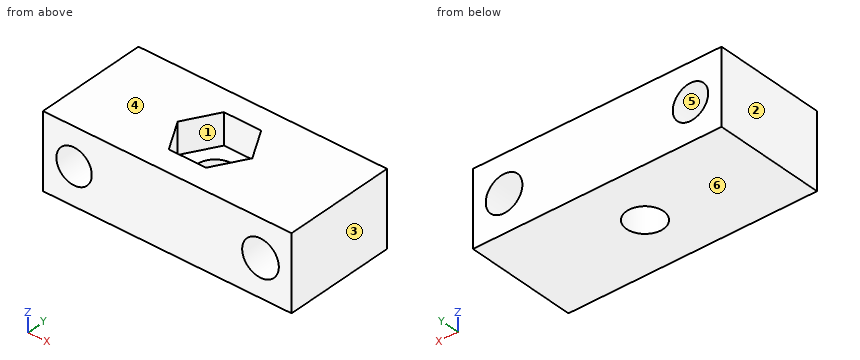
Autodesk Inventor part; units mm, degrees
ref_plane "YZ Plane" through (0, 0, 0) normal (1, 0, 0) x (0, 1, 0)
ref_plane "XZ Plane" through (0, 0, 0) normal (0, 1, 0) x (-1, 0, 0)
ref_plane "XY Plane" through (0, 0, 0) normal (0, 0, 1) x (1, 0, 0)
sketch "Sketch1" plane through (0, 0, 0) normal (0, 1, 0) x (-1, 0, 0)
  line L0 (0, 0) -> (40, 0)
  line L1 (40, 0) -> (40, -12)
  line L2 (40, -12) -> (0, -12)
  line L3 (0, -12) -> (0, 0)
  circle A0 centre (35, -6) radius 2.85
  circle A1 centre (5, -6) radius 2.95
  dimension "d0" = 40
  dimension "d1" = 12
  dimension "d2" = 5.7
  dimension "d3" = 5.9
  dimension "d4" = 5
  dimension "d6" = 6
  dimension "d33" = 5
extrude "Extrusion1" add sketch "Sketch1" along normal blind 18
sketch "Sketch8" plane through (-40, 0, 0) normal (0, 0, 1) x (1, 0, 0)
  circle A0 centre (20, 9) radius 2.95
  line L0 (0, 0) -> (0, 18)
  line L1 (40, 0) -> (0, 0)
  dimension "d34" = 5.9
  dimension "d35" = 20
  dimension "d36" = 9
extrude "Extrusion8" cut sketch "Sketch8" against normal up to next
sketch "Sketch9" plane through (-40, 0, 0) normal (0, 0, 1) x (1, 0, 0)
  circle A0 centre (20, 9) radius 2.95
  line L0 (16.9978, 3.8) -> (13.9956, 9)
  line L1 (13.9956, 9) -> (16.9978, 14.2)
  line L2 (16.9978, 14.2) -> (23.0022, 14.2)
  line L3 (23.0022, 14.2) -> (26.0044, 9)
  line L4 (26.0044, 9) -> (23.0022, 3.8)
  line L5 (23.0022, 3.8) -> (16.9978, 3.8)
  line L6 (40, 0) -> (0, 0)
  dimension "d39" = 10.4
extrude "Extrusion9" cut sketch "Sketch9" against normal blind 5
properties part number "back_sprocket_holder"
Input: part model. Units: mm. Frame: model coordinates. Face numbers are marked on the shaded views. A direction names the side the tool comes from. Give positions to 0.01 mm unless a question says otherwise; leave off trailing zeros. Loops run counter-clockwise (first coordinate to the right, second up) from the corner with the lowest first, then second, coordinate; pieces in that order, holes last. Notation, with made-up numbers: (-22.5, 2.5) -> (-0.5, 2.5) arc R20 ccw to (-0.5, 37.5) -> close; hole circle Ø1 at (-1, -2.5). An arc over 180 degrees is marked (long way). Use a Markdown table: item, result.
Q1. Section query B-B, the plane y = 10.75. Return the cut outline in (x, z), plus the area to 3 significant figures.
Entries:
| item | result |
|---|---|
| outline | (-40, -12) -> (-22.37, -12) -> (-22.37, -5) -> (-24.99, -5) -> (-24.99, 0) -> (-40, 0) -> close; (-17.63, -12) -> (0, -12) -> (0, 0) -> (-15.01, 0) -> (-15.01, -5) -> (-17.63, -5) -> close; hole circle Ø5.7 at (-35, -6); hole circle Ø5.9 at (-5, -6) |
| area | 344 mm² |
Q2. Pull-direction query (Z, two-part tool) for the marked faces 3, 4, 5 and 6; classes: pulls with the +Z half, pulls with the -Z half, needs draft (parallel to the pull), parting line crosses it, or undercut.
Entries:
| item | result |
|---|---|
| face 3 | needs draft |
| face 4 | pulls with the +Z half |
| face 5 | undercut |
| face 6 | pulls with the -Z half |
Q3. Section query D-D, the plane y = 15.25. Return the cut outline in (x, z), plus the area to 3 significant figures.
Entries:
| item | result |
|---|---|
| outline | (-40, -12) -> (0, -12) -> (0, 0) -> (-40, 0) -> close; hole circle Ø5.7 at (-35, -6); hole circle Ø5.9 at (-5, -6) |
| area | 427 mm² |
Q4. Access query for the marked faces 1 and 2. Directions: +Z, -Z, +X, -X, +Y, -Y. A direction counts if a zero-diameter tool reaches every point of the face in a straight line with its end or side. Return the directions, or none.
Entries:
| item | result |
|---|---|
| face 1 | +Z |
| face 2 | +Z, -Z, -X, +Y, -Y |
Q5. Section query A-A, the plane x = -35. Return the cut outline in (y, z).
Entries:
| item | result |
|---|---|
| outline | (0, -12) -> (18, -12) -> (18, -8.85) -> (0, -8.85) -> close; (0, -3.15) -> (18, -3.15) -> (18, 0) -> (0, 0) -> close |
Q6. Ray query, probe 1 along Z at (x, y) = (-35, 7.5); probe 2 along Y at (x, z) = (-22, -4.5); probe 3 along X at (y, z) = (16.75, -4). Return the intervals inside material, ascending. Write a range as from..to.
Entries:
| item | result |
|---|---|
| probe 1 | z = -12..-8.85, -3.15..0 |
| probe 2 | y = 0..3.8, 14.2..18 |
| probe 3 | x = -40..-37.03, -32.97..-7.17, -2.83..0 |
Q7. First-contact query: P1, Ø3, axis at x = -20, y = 10.5, coming from the +Z side. Flat tip, straight axial feed; report the tip coordinate or a pass-through.
Entries:
| item | result |
|---|---|
| P1 | stops at z = -5 |
Q8. Section query C-C, the plane z = -0.75. Return the cut outline in (x, y).
Entries:
| item | result |
|---|---|
| outline | (-40, 0) -> (0, 0) -> (0, 18) -> (-40, 18) -> close; hole (-26, 9) -> (-23, 3.8) -> (-17, 3.8) -> (-14, 9) -> (-17, 14.2) -> (-23, 14.2) -> close |
